Check sheet for the modelled part. Datum: model origin and axes. Units: mm. A direction names the side the tool comes from. Round coordinates to 2 decimals unless told otherwise and drop trailing zeros. Write each loop counter-clockwise with the first axis right and the second up, starting at its lowest first coordinate (ties: lowest second). Pieces come first, ordered by that corner, then holes. Notation, with made-up numbers: M 74,39 L 109,39 A16 cw 109,63 Z; hole C 20,18 d7. An arc over 180 degrees is marked long. Answer in a Markdown table with one row per item.
```python
from build123d import *

# Parameters (mm, degrees)
SKETCH1_W               = 60
SKETCH1_H               = 22
SKETCH1_R               = 2.15
BOSS_EXTRUDE1_DEPTH     = 4
SKETCH2_R               = 1.7
BOSS_EXTRUDE2_DEPTH     = 9
CUT_EXTRUDE1_DEPTH      = 34
MIRROR5_COPY_1_SKETCH_R = 1.7
MIRROR5_COPY_1_DEPTH    = 9
MIRROR5_COPY_2_DEPTH    = 34
FILLET1_START           = -11.0000001
FILLET1_DEPTH           = 9.0000001
FILLET1_START_2         = 2
FILLET1_2_DEPTH         = 9
FILLET1_START_3         = 4
FILLET1_3_OUTLINE_R     = 2.15
FILLET1_3_DEPTH         = 4.037755723
FILLET1_START_4         = -30
FILLET1_4_DEPTH         = 60


with BuildPart() as part:
    # Sketch1 → Boss-Extrude1 (new body)
    with BuildSketch(Plane(origin=(0, 0, 0), x_dir=(1, 0, 0), z_dir=(0, 1, 0))):
        Rectangle(SKETCH1_W, SKETCH1_H)
        with Locations(Location((-18, 5, 0), (0, 0, 270))):
            Circle(SKETCH1_R, mode=Mode.SUBTRACT)
        with Locations(Location((-18, -5, 0), (0, 0, 270))):
            Circle(SKETCH1_R, mode=Mode.SUBTRACT)
        with Locations(Location((18, 5, 0), (0, 0, 90))):
            Circle(SKETCH1_R, mode=Mode.SUBTRACT)
        with Locations(Location((18, -5, 0), (0, 0, 90))):
            Circle(SKETCH1_R, mode=Mode.SUBTRACT)
    extrude(amount=BOSS_EXTRUDE1_DEPTH)

    # Sketch2 → Boss-Extrude2 (add)
    with BuildSketch(Plane.XY.offset(2)):
        with BuildLine():
            Line((-30, 4), (-31.048991933, 8.037755723))
            ThreePointArc((-31.048991933, 8.037755723), (-26.5, 13.919564671), (-21.951008067, 8.037755723))
            Line((-21.951008067, 8.037755723), (-23, 4))
            Line((-23, 4), (-30, 4))
        make_face()
        with Locations((-26.5, 9.219564671)):
            Circle(SKETCH2_R, mode=Mode.SUBTRACT)
    boss_extrude2 = extrude(amount=BOSS_EXTRUDE2_DEPTH)

    # Sketch3 → Cut-Extrude1 (cut)
    with BuildSketch(Plane(origin=(0, 0, 0), x_dir=(0, 0, -1), z_dir=(1, 0, 0))):
        Polygon((-5, 13.919564671), (-11, 4), (-11, 13.919564671), align=None)
    cut_extrude1 = extrude(amount=-CUT_EXTRUDE1_DEPTH, mode=Mode.SUBTRACT)

    # Mirror4: Boss-Extrude2, Cut-Extrude1 across plane
    add(boss_extrude2.mirror(Plane.XY))
    add(cut_extrude1.mirror(Plane.XY), mode=Mode.SUBTRACT)

    # Mirror5: Boss-Extrude2, Cut-Extrude1 across plane
    add(boss_extrude2.mirror(Plane(origin=(0, 0, 0), x_dir=(0, 0, 1), z_dir=(1, 0, 0))))
    add(cut_extrude1.mirror(Plane(origin=(0, 0, 0), x_dir=(0, 0, 1), z_dir=(1, 0, 0))), mode=Mode.SUBTRACT)

    # Mirror5 copy 1 sketch → Mirror5 copy 1 (add)
    with BuildSketch(Plane(origin=(0, 0, -2), x_dir=(-1, 0, 0), z_dir=(0, 0, -1))):
        with BuildLine():
            Line((-30, 4), (-31.048991933, 8.037755723))
            ThreePointArc((-31.048991933, 8.037755723), (-26.5, 13.919564671), (-21.951008067, 8.037755723))
            Line((-21.951008067, 8.037755723), (-23, 4))
            Line((-23, 4), (-30, 4))
        make_face()
        with Locations((-26.5, 9.219564671)):
            Circle(MIRROR5_COPY_1_SKETCH_R, mode=Mode.SUBTRACT)
    extrude(amount=MIRROR5_COPY_1_DEPTH)

    # Mirror5 copy 2 sketch → Mirror5 copy 2 (cut)
    with BuildSketch(Plane.ZY):
        Polygon((-5, 13.919564671), (-11, 4), (-11, 13.919564671), align=None)
    extrude(amount=-MIRROR5_COPY_2_DEPTH, mode=Mode.SUBTRACT)

    # Fillet1: read off the stored shape, not the designer's step
    # Fillet1 outline → Fillet1 (add)
    with BuildSketch(Plane.XY.offset(FILLET1_START)):
        with BuildLine():
            ThreePointArc((21.951008067, 8.037755723), (21.80348703, 9.400578254), (22.055466759, 10.748003177))
            ThreePointArc((22.055466759, 10.748003177), (18.407628714, 5.859976406), (12.599013054, 4))
            Line((12.599013054, 4), (23, 4))
            Line((23, 4), (21.951008067, 8.037755723))
        make_face()
        with BuildLine():
            Line((-23, 4), (-12.599013054, 4))
            ThreePointArc((-12.599013054, 4), (-18.407628714, 5.859976406), (-22.055466759, 10.748003177))
            ThreePointArc((-22.055466759, 10.748003177), (-21.80348703, 9.400578254), (-21.951008067, 8.037755723))
            Line((-21.951008067, 8.037755723), (-23, 4))
        make_face()
    extrude(amount=FILLET1_DEPTH)

    # Fillet1 2 outline → Fillet1 2 (add)
    with BuildSketch(Plane.XY.offset(FILLET1_START_2)):
        with BuildLine():
            ThreePointArc((21.951008067, 8.037755723), (21.80348703, 9.400578254), (22.055466759, 10.748003177))
            ThreePointArc((22.055466759, 10.748003177), (18.407628714, 5.859976406), (12.599013054, 4))
            Line((12.599013054, 4), (23, 4))
            Line((23, 4), (21.951008067, 8.037755723))
        make_face()
        with BuildLine():
            Line((-23, 4), (-12.599013054, 4))
            ThreePointArc((-12.599013054, 4), (-18.407628714, 5.859976406), (-22.055466759, 10.748003177))
            ThreePointArc((-22.055466759, 10.748003177), (-21.80348703, 9.400578254), (-21.951008067, 8.037755723))
            Line((-21.951008067, 8.037755723), (-23, 4))
        make_face()
    extrude(amount=FILLET1_2_DEPTH)

    # Fillet1 3 outline → Fillet1 3 (cut)
    with BuildSketch(Plane(origin=(0, 0, 0), x_dir=(1, 0, 0), z_dir=(0, 1, 0)).offset(FILLET1_START_3)):
        with Locations((-18, -5)):
            Circle(FILLET1_3_OUTLINE_R)
        with Locations((-18, 5)):
            Circle(FILLET1_3_OUTLINE_R)
        with Locations((18, 5)):
            Circle(FILLET1_3_OUTLINE_R)
        with Locations((18, -5)):
            Circle(FILLET1_3_OUTLINE_R)
    extrude(amount=FILLET1_3_DEPTH, mode=Mode.SUBTRACT)

    # Fillet1 4 outline → Fillet1 4 (cut)
    with BuildSketch(Plane.YZ.offset(FILLET1_START_4)):
        Polygon((12, 11), (4, 11), (12, 6.161077971), align=None)
        Polygon((12, -11), (12, -6.161077971), (4, -11), align=None)
    extrude(amount=FILLET1_4_DEPTH, mode=Mode.SUBTRACT)


solid = part.part
```
1. Access from +Z, -Z, +X, -X, +Y, -Y to the whole of each face (thin tool, end or side, straight path). Record for faces 1 (the face through (18.48, 5.91, 7.44)), 2 (the face through (0, 4, 0)), 3 (the face through (26, 7, 2)).
Found:
| item | result |
|---|---|
| face 1 | +Z, -Z, +Y |
| face 2 | +Y |
| face 3 | +X, -X, +Y |
2. Section check B-B, the plane y = 13. Record the cut outline in (x, z), and give its area (3 significant figures).
Found:
| item | result |
|---|---|
| outline | M -29.29,-5.56 L -23.71,-5.56 L -23.71,-2 L -29.29,-2 Z; M -29.29,2 L -23.71,2 L -23.71,5.56 L -29.29,5.56 Z; M 23.71,-5.56 L 29.29,-5.56 L 29.29,-2 L 23.71,-2 Z; M 23.71,2 L 29.29,2 L 29.29,5.56 L 23.71,5.56 Z |
| area | 79.4 mm2 |
3. Section check D-D, the plane x = 7.5. Record the cut outline in (y, z).
Found:
| item | result |
|---|---|
| outline | M 0,-11 L 4,-11 L 4,11 L 0,11 Z |
4. Section check C-C, the plane x = -26.5. Record the cut outline in (y, z).
Found:
| item | result |
|---|---|
| outline | M 0,-11 L 4,-11 L 7.52,-8.87 L 7.52,-2 L 4,-2 L 4,2 L 7.52,2 L 7.52,8.87 L 4,11 L 0,11 Z; M 10.92,-6.81 L 13.92,-5 L 13.92,-2 L 10.92,-2 Z; M 10.92,2 L 13.92,2 L 13.92,5 L 10.92,6.81 Z |
5. Section check A-A, the plane z = -4. Record the cut outline in (x, y), and give its area (3 significant figures).
Found:
| item | result |
|---|---|
| outline | M -31.05,8.04 L -30,4 L -30,0 L -19.9,0 L -19.9,7.17 A10 cw -22.06,10.75 A4.7 ccw Z; M -16.1,0 L 16.1,0 L 16.1,4.63 A10 cw 12.6,4 L -12.6,4 A10 cw -16.1,4.63 Z; M 19.9,0 L 30,0 L 30,4 L 31.05,8.04 A4.7 ccw 22.06,10.75 A10 cw 19.9,7.17 Z; hole C -26.5,9.22 d3.4; hole C 26.5,9.22 d3.4 |
| area | 372 mm2 |
6. Draft check along Y on faces 4 (the face through (30.517, 5.991, 5.437)), 5 (the face through (-29.36, 12.95, -3.78)), 6 (the face through (26.87, 7.56, 4.62)). Enter one of: +Y half, -Y half, draft (parallel to the pull), parting line (faces both ways), or undercut.
Found:
| item | result |
|---|---|
| face 4 | -Y half |
| face 5 | parting line |
| face 6 | undercut |
7. Scan lines: L1, parallel to X at y = 2.25, z = 5; L2, parallel to Z at x = -18, y = 2.5; L3, parallel to X at y = 1, z = 5.75. Record each from-to range of solid material in increasing order.
Found:
| item | result |
|---|---|
| L1 | x = -30 to -20.15, -15.85 to 15.85, 20.15 to 30 |
| L2 | z = -11 to -7.15, -2.85 to 2.85, 7.15 to 11 |
| L3 | x = -30 to -20.01, -15.99 to 15.99, 20.01 to 30 |
8. Go/stop test with flat-tipped pins: pin 1 (3 mm diameter, centred on x = -20, y = 9.5, fed in from +Z); pin 2 (5.5 mm diameter, centred on x = -18, z = 5, fed in from +Y); pin 3 (3 mm diameter, centred on x = 7.5, z = -1.5, fed in from +Y). Record where each tip stops, or that it passes through.
Found:
| item | result |
|---|---|
| pin 1 | stops at z = 8.46 |
| pin 2 | stops at y = 8.21 |
| pin 3 | stops at y = 4 |
